from build123d import *

# Parameters (mm, degrees)
SKIZZE1_W                       = 37.5
SKIZZE1_H                       = 33
AUFSATZ_LINEAR_AUSTRAGEN1_DEPTH = 2.5
SKIZZE2_W                       = 3
SKIZZE2_H                       = 33
SKIZZE2_W_2                     = 8
SKIZZE2_H_2                     = 5.1
AUFSATZ_LINEAR_AUSTRAGEN2_DEPTH = 12.3
SCHNITT_LINEAR_AUSTRAGEN3_DEPTH = 30.031922086
SKIZZE5_R                       = 1.2
SCHNITT_LINEAR_AUSTRAGEN4_DEPTH = 42.006584837
SKIZZE7_R                       = 1.05
SCHNITT_LINEAR_AUSTRAGEN5_DEPTH = 10


with BuildPart() as part:
    # Skizze1 → Aufsatz-Linear austragen1 (new body)
    with BuildSketch(Plane(origin=(0, 0, 0), x_dir=(1, 0, 0), z_dir=(0, 1, 0))):
        Rectangle(SKIZZE1_W, SKIZZE1_H)
    extrude(amount=AUFSATZ_LINEAR_AUSTRAGEN1_DEPTH)

    # Skizze2 → Aufsatz-Linear austragen2 (add)
    with BuildSketch(Plane(origin=(0, 2.5, 0), x_dir=(1, 0, 0), z_dir=(0, 1, 0))):
        with Locations((-17.25, 0)):
            Rectangle(SKIZZE2_W, SKIZZE2_H)
        with Locations((0.75, -13.95)):
            Rectangle(SKIZZE2_W_2, SKIZZE2_H_2)
        with Locations((0.75, 13.95)):
            Rectangle(SKIZZE2_W_2, SKIZZE2_H_2)
    extrude(amount=AUFSATZ_LINEAR_AUSTRAGEN2_DEPTH)

    # Skizze6 → Schnitt-Linear austragen3 (cut, through all)
    with BuildSketch(Plane.XZ):
        with BuildLine():
            ThreePointArc((-10.291545894, -1.098445774), (-9.551783389, -0.756868708), (-9.25, 0))
            ThreePointArc((-9.25, 0), (-9.551783389, 0.756868708), (-10.291545894, 1.098445774))
            ThreePointArc((-10.291545894, 1.098445774), (-10.35, 0), (-10.291545894, -1.098445774))
        make_face()
        with BuildLine():
            ThreePointArc((-10.291545894, -1.098445774), (-10.35, 0), (-10.291545894, 1.098445774))
            ThreePointArc((-10.291545894, 1.098445774), (-11.45, 0), (-10.291545894, -1.098445774))
        make_face()
        with BuildLine():
            ThreePointArc((-1.098445774, 10.291545894), (0, 9.25), (1.098445774, 10.291545894))
            ThreePointArc((1.098445774, 10.291545894), (0, 10.35), (-1.098445774, 10.291545894))
        make_face()
        with BuildLine():
            ThreePointArc((-1.098445774, 10.291545894), (0, 10.35), (1.098445774, 10.291545894))
            ThreePointArc((1.098445774, 10.291545894), (1.099611375, 10.320762617), (1.1, 10.35))
            ThreePointArc((1.1, 10.35), (-0.029237383, 11.449611375), (-1.098445774, 10.291545894))
        make_face()
        with BuildLine():
            ThreePointArc((10.291545894, -1.098445774), (11.106868708, -0.798216611), (11.45, 0))
            ThreePointArc((11.45, 0), (11.106868708, 0.798216611), (10.291545894, 1.098445774))
            ThreePointArc((10.291545894, 1.098445774), (10.35, 0), (10.291545894, -1.098445774))
        make_face()
        with BuildLine():
            ThreePointArc((10.291545894, -1.098445774), (10.35, 0), (10.291545894, 1.098445774))
            ThreePointArc((10.291545894, 1.098445774), (9.25, 0), (10.291545894, -1.098445774))
        make_face()
        with BuildLine():
            ThreePointArc((-1.098445774, -10.291545894), (-0.029237383, -11.449611375), (1.1, -10.35))
            ThreePointArc((1.1, -10.35), (1.099611375, -10.320762617), (1.098445774, -10.291545894))
            ThreePointArc((1.098445774, -10.291545894), (0, -10.35), (-1.098445774, -10.291545894))
        make_face()
        with BuildLine():
            ThreePointArc((-1.098445774, -10.291545894), (0, -10.35), (1.098445774, -10.291545894))
            ThreePointArc((1.098445774, -10.291545894), (0, -9.25), (-1.098445774, -10.291545894))
        make_face()
    extrude(amount=-SCHNITT_LINEAR_AUSTRAGEN3_DEPTH, mode=Mode.SUBTRACT)

    # Skizze5 → Schnitt-Linear austragen4 (cut, through all)
    with BuildSketch(Plane(origin=(-15.75, 0, 0), x_dir=(0, 0, -1), z_dir=(1, 0, 0))):
        with Locations((5.7, 8.65)):
            Circle(SKIZZE5_R)
    extrude(amount=-SCHNITT_LINEAR_AUSTRAGEN4_DEPTH, mode=Mode.SUBTRACT)

    # Skizze7 → Schnitt-Linear austragen5 (cut)
    with BuildSketch(Plane(origin=(4.75, 0, 0), x_dir=(0, 0, -1), z_dir=(1, 0, 0))):
        with Locations((-14.35, 8.65)):
            Circle(SKIZZE7_R)
        with Locations((14.35, 8.65)):
            Circle(SKIZZE7_R)
    extrude(amount=-SCHNITT_LINEAR_AUSTRAGEN5_DEPTH, mode=Mode.SUBTRACT)


solid = part.part
The model under review builds one solid part; all positions refer to its coordinate system, in mm. A direction names the side the tool comes from. Coordinates: 2 decimals unless noted, no trailing zeros. Write each loop counter-clockwise with the first axis right and the second up, starting at its lowest first coordinate (ties: lowest second). Pieces come first, ordered by that corner, then holes. Notation, with made-up numbers: (56, -21) - (86, -21) arc R19 cw to (86, -10) - close; hole circle Ø7 at (32, 66.25). An arc over 180 degrees is marked (long way). Answer as CSV lines item,"result".
(1) We need section B-B (z = 14.35). Give the boundary of the cut face in (x, y).
Data:
outline,"(-18.75, 0) - (18.75, 0) - (18.75, 2.5) - (4.75, 2.5) - (4.75, 7.6) - (-3.25, 7.6) - (-3.25, 2.5) - (-15.75, 2.5) - (-15.75, 14.8) - (-18.75, 14.8) - close; (-3.25, 9.7) - (4.75, 9.7) - (4.75, 14.8) - (-3.25, 14.8) - close"
(2) Clearance check with flat-ended pins moving along their axes: pin 1 Ø6 at (y, z) = (11.5, 0.5) entering from +X; pin 2 Ø6 at (x, z) = (-3.5, -2) entering from +Y; pin 3 Ø5.5 at (y, z) = (7, 13) entering from +X. State where each tip first meets the part, or that it passes through.
Data:
pin 1,"stops at x = -15.75"
pin 2,"stops at y = 2.5"
pin 3,"stops at x = 4.75"
(3) We need section C-C (y = 11.5). Give the boundary of the cut face in (x, z).
Data:
outline,"(-18.75, -16.5) - (-15.75, -16.5) - (-15.75, 16.5) - (-18.75, 16.5) - close; (-3.25, -16.5) - (4.75, -16.5) - (4.75, -11.4) - (0.33, -11.4) arc R1.1 cw to (-0.33, -11.4) - (-3.25, -11.4) - close; (-3.25, 11.4) - (-0.33, 11.4) arc R1.1 cw to (0.33, 11.4) - (4.75, 11.4) - (4.75, 16.5) - (-3.25, 16.5) - close"
(4) Tool access review of faces 4 (the flat face through (-2, 9, -11.4)), 5 (the flat face through (-3.25, 9, 13)), 6 (the cylindrical face through (0.8, 8.2, -15.3)): name each direction out of +Z, -Z, +X, -X, +Y, -Y from which nothing blocks a thin tool from reaching the whole face with its end or side.
Data:
face 4,"+X, +Y"
face 5,"+Z, -Z, +Y"
face 6,"+X"
(5) For line 1 along X through (y, z) = (10.25, -11.5); line 2 along Y through (x, z) = (0.5, 14.35); line 3 along Y through (x, z) = (-17.25, -5.7), list the stretches that pass through material, from the lowest coordinate up. Write a range as [from, to].
Data:
line 1,"x = [-18.75, -15.75], [-3.25, 4.75]"
line 2,"y = [0, 7.6], [9.7, 14.8]"
line 3,"y = [0, 7.45], [9.85, 14.8]"
(6) We need section A-A (y = 8.65). Give the boundary of the cut face in (x, z), plus the area to 3 significant figures.
Data:
outline,"(-18.75, -16.5) - (-15.75, -16.5) - (-15.75, -6.9) - (-18.75, -6.9) - close; (-18.75, -4.5) - (-15.75, -4.5) - (-15.75, 16.5) - (-18.75, 16.5) - close; (-3.25, -16.5) - (4.75, -16.5) - (4.75, -15.4) - (-3.25, -15.4) - close; (-3.25, -13.3) - (4.75, -13.3) - (4.75, -11.4) - (0.33, -11.4) arc R1.1 cw to (-0.33, -11.4) - (-3.25, -11.4) - close; (-3.25, 11.4) - (-0.33, 11.4) arc R1.1 cw to (0.33, 11.4) - (4.75, 11.4) - (4.75, 13.3) - (-3.25, 13.3) - close; (-3.25, 15.4) - (4.75, 15.4) - (4.75, 16.5) - (-3.25, 16.5) - close"
area,"140 mm2"
(7) We need section D-D (x = -12). Give the boundary of the cut face in (y, z), plus the area to 3 significant figures.
Data:
outline,"(0, -16.5) - (2.5, -16.5) - (2.5, 16.5) - (0, 16.5) - close"
area,"82.5 mm2"
(8) Mouldability with a two-part tool opening along Z and no side actions: class faces 1 (the flat face through (4.75, 9, -13)), 2 (the flat face through (0, 6, -16.5)), 3 (the cylindrical face through (0.8, 8.7, 15.4)) as pulls with the +Z half, pulls with the -Z half, needs draft (parallel to the pull), parting line crosses it, or undercut.
Data:
face 1,"needs draft"
face 2,"pulls with the -Z half"
face 3,"undercut"
